Geometry check sheet. Reference: the model listing, model coordinates, mm. Face numbers are marked on the shaded views. A direction names the side the tool comes from. Round coordinates to 2 decimals unless told otherwise and drop trailing zeros. Write each loop counter-clockwise with the first axis right and the second up, starting at its lowest first coordinate (ties: lowest second). Pieces come first, ordered by that corner, then holes. Notation, with made-up numbers: (-2.5, -39) -> (49.5, -39) arc R36 cw to (49.5, 0) -> close; hole circle Ø8 at (-31, 32.5). An arc over 180 degrees is marked (long way). One line per question, with ' | ' between items.
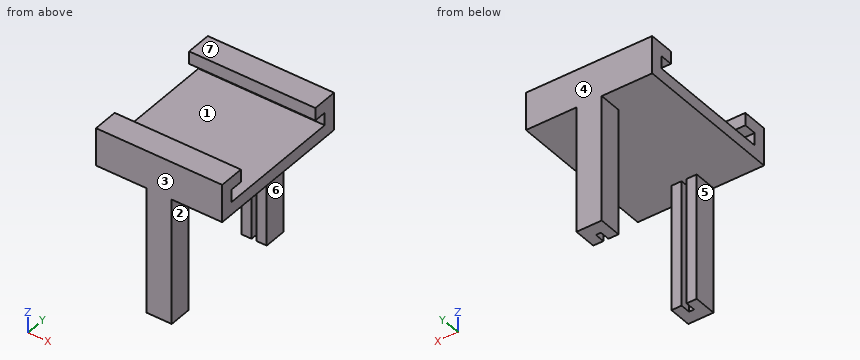
Autodesk Inventor part; units mm, degrees
ref_plane "YZ Plane" through (0, 0, 0) normal (1, 0, 0) x (0, 1, 0)
ref_plane "XZ Plane" through (0, 0, 0) normal (0, 1, 0) x (-1, 0, 0)
ref_plane "XY Plane" through (0, 0, 0) normal (0, 0, 1) x (1, 0, 0)
sketch "Sketch1" plane through (0, 0, 0) normal (0, 0, 1) x (1, 0, 0)
  line L0 (-25, 30) -> (25, 30)
  line L1 (25, 30) -> (25, -30)
  line L2 (25, -30) -> (-25, -30)
  line L3 (-25, -30) -> (-25, 30)
  point P0 (0, 0)
  dimension "d0" = 50
  dimension "d1" = 60
  dimension "d2" = 30
  dimension "d3" = 25
extrude "Extrusion1" add sketch "Sketch1" along normal blind 5
sketch "Sketch2" plane through (0, 0, 5) normal (0, 0, 1) x (1, 0, 0)
  line L0 (-25, 30) -> (-25, -30)
  line L1 (-25, 25) -> (25, 25)
  line L2 (25, -30) -> (25, 30)
  line L3 (25, 30) -> (-25, 30)
  point P0 (0, 0)
  dimension "d6" = 5
extrude "Extrusion2" add sketch "Sketch2" along normal blind 10
sketch "Sketch3" plane through (0, 0, 5) normal (0, 0, 1) x (1, 0, 0)
  line L0 (-25, -30) -> (-25, 30)
  line L1 (-25, -25) -> (25, -25)
  line L2 (25, 30) -> (25, -30)
  line L3 (-25, -30) -> (25, -30)
  point P0 (0, 0)
  dimension "d9" = 5
extrude "Extrusion3" add sketch "Sketch3" along normal blind 10
sketch "Sketch4" plane through (-25, -25, 5) normal (0, 1, 0) x (1, 0, 0)
  line L0 (0, 5) -> (0, -10)
  line L1 (0, -5) -> (50, -5)
  line L2 (50, 5) -> (50, -10)
  line L3 (0, -10) -> (50, -10)
  point P0 (25, 5)
  dimension "d12" = 5
extrude "Extrusion4" add sketch "Sketch4" along normal blind 5
sketch "Sketch5" plane through (-25, 25, 5) normal (0, -1, 0) x (1, 0, 0)
  line L0 (0, -5) -> (0, 10)
  line L1 (0, 5) -> (50, 5)
  line L2 (50, -5) -> (50, 10)
  line L3 (50, 10) -> (0, 10)
  point P0 (25, -5)
  dimension "d15" = 5
extrude "Extrusion5" add sketch "Sketch5" along normal blind 5
sketch "Sketch12" plane through (0, 0, 0) normal (0, 0, -1) x (-1, 0, 0)
  line L0 (25, 30) -> (-25, 30)
  line L1 (-5, 30) -> (5, 30)
  line L2 (5, 30) -> (5, 25)
  line L3 (5, 25) -> (-5, 25)
  line L4 (-5, 25) -> (-5, 30)
  line L5 (-25, 30) -> (-25, -30)
  line L6 (-5, 25) -> (-1, 25)
  line L7 (-1, 25) -> (-1, 21)
  line L8 (-1, 21) -> (-5, 21)
  line L9 (-5, 21) -> (-5, 25)
  line L10 (5, 25) -> (1, 25)
  line L11 (1, 25) -> (1, 21)
  line L12 (1, 21) -> (5, 21)
  line L13 (5, 21) -> (5, 25)
  point P0 (0, 0)
  dimension "d42" = 10
  dimension "d43" = 5
  dimension "d44" = 20
  dimension "d45" = 4
  dimension "d46" = 4
  dimension "d47" = 4
  dimension "d50" = 4
extrude "Extrusion12" add sketch "Sketch12" along normal blind 50
mirror "Mirror1" about plane through (0, 0, 0) normal (0, 1, 0) of "Extrusion12"
properties part number "Substrategrip90degreesThick"
(1) Sectioned sample at D-D on z = 8.5. Record the cut outline in (x, y), then the cut area to 3 significant figures.
Resolved:
outline: (-25, -30) -> (25, -30) -> (25, -25) -> (-25, -25) -> close; (-25, 25) -> (25, 25) -> (25, 30) -> (-25, 30) -> close | area: 500 mm2
(2) Access from +Z, -Z, +X, -X, +Y, -Y to the whole of each face (thin tool, end or side, straight path). Record for the marked faces 5, 6 and 7.
Resolved:
face 5: -Z, -X, +Y, -Y | face 6: -Z, +X, +Y, -Y | face 7: +Z, +X, -X, +Y, -Y
(3) Go/stop test with flat-tipped pins: pin 1 (7 mm diameter, centred on y = -26.5, z = -18.5, fed in from -X); pin 2 (4.5 mm diameter, centred on y = -26, z = -26.5, fed in from +X); pin 3 (5 mm diameter, centred on x = 16, y = -6.5, fed in from -Z). Record where each tip stops, or that it passes through.
Resolved:
pin 1: stops at x = -5 | pin 2: stops at x = 5 | pin 3: stops at z = 0
(4) Material ranges on line 1 (Z direction, x = -18.5, y = -21.5); line 2 (X direction, y = -24.5, z = -5); line 3 (Z direction, x = -19, y = -11.5), recorded low to high.
Resolved:
line 1: z = 0 to 5, 10 to 15 | line 2: x = -5 to -1, 1 to 5 | line 3: z = 0 to 5
(5) Sectioned sample at B-B on z = -28. Record the cut outline in (x, y), then the cut area to 3 significant figures.
Resolved:
outline: (-5, -30) -> (5, -30) -> (5, -21) -> (1, -21) -> (1, -25) -> (-1, -25) -> (-1, -21) -> (-5, -21) -> close; (-5, 21) -> (-1, 21) -> (-1, 25) -> (1, 25) -> (1, 21) -> (5, 21) -> (5, 30) -> (-5, 30) -> close | area: 164 mm2
(6) Draft check along Y on the marked faces 1, 2, 3 and 4. Enter one of: +Y half, -Y half, draft (parallel to the pull), parting line (faces both ways), or undercut.
Resolved:
face 1: undercut | face 2: draft | face 3: -Y half | face 4: +Y half
(7) Sectioned sample at C-C on x = -11.5. Record the cut outline in (y, z).
Resolved:
outline: (-30, 0) -> (30, 0) -> (30, 15) -> (20, 15) -> (20, 10) -> (25, 10) -> (25, 5) -> (-25, 5) -> (-25, 10) -> (-20, 10) -> (-20, 15) -> (-30, 15) -> close
(8) Sectioned sample at A-A on y = 23.5. Record the cut outline in (x, z), then the cut area to 3 significant figures.
Resolved:
outline: (-25, 0) -> (-5, 0) -> (-5, -50) -> (-1, -50) -> (-1, 0) -> (1, 0) -> (1, -50) -> (5, -50) -> (5, 0) -> (25, 0) -> (25, 5) -> (-25, 5) -> close; (-25, 10) -> (25, 10) -> (25, 15) -> (-25, 15) -> close | area: 900 mm2
